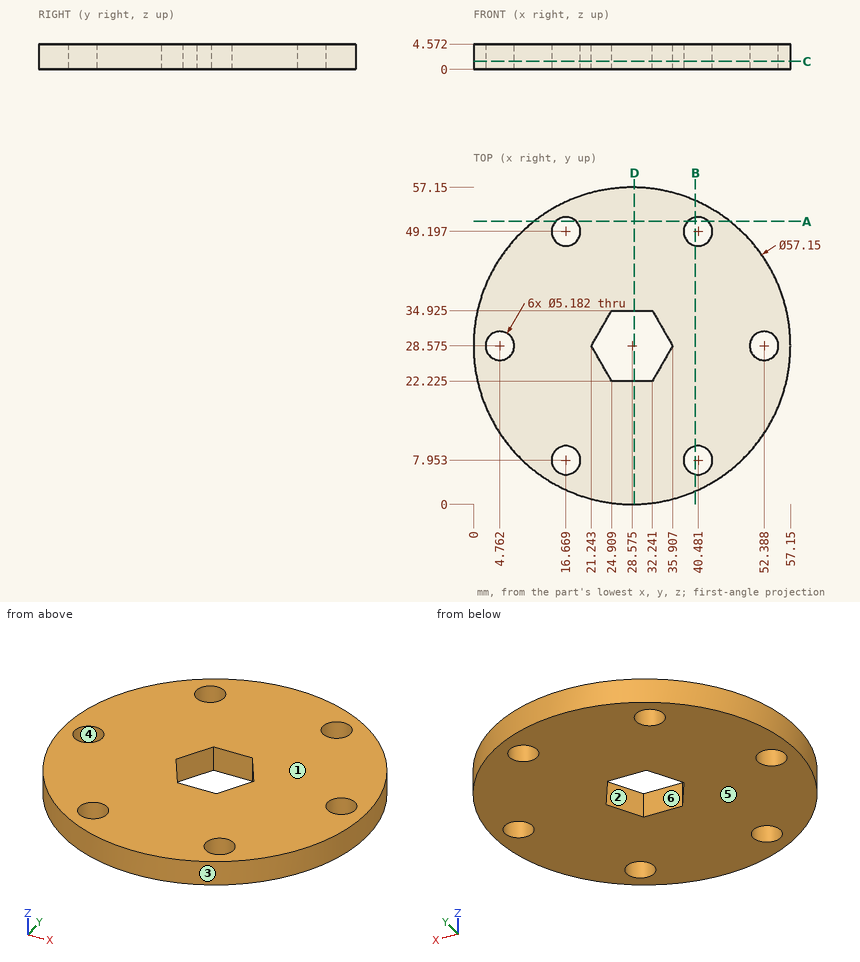
Can you work these out from the drawing? Everything is in mm from the part's minimum corner. A direction names the side the tool comes from. Give positions to 0.01 mm unless a question says otherwise; leave off trailing zeros. Order: outer loops, then holes, each group sorted by start corner. A loop starts at its lowest first (then second) coordinate and runs counter-clockwise, first axis right, second up.
Item 1: If we section it at B-B, the plane x = 40: Write out the boundary of the cut face in (y, z), plus the area to 3 significant figures.
Item 2: If we section it at C-C, the plane z = 1.45: Count the separate pieces of the cut face and the enclosed holes in it, plus the area to 3 significant figures.
Item 3: If we section it at D-D, the plane x = 29: Write out the boundary of the cut face in (y, z) (1 decimal).
Item 4: If we section it at A-A, the plane y = 51: Write out the boundary of the cut face in (x, z) (1 decimal), plus the area to 3 significant figures.
Item 5: For the marked faces 5 and 6, which set-ups out of +Z, -Z, +X, -X, +Y, -Y let a thin tool reach every point of the face, with its end or its side?
Item 6: If we mould it in two halves opening along Y, with no side actions, what happens to the marked faces 1, 2, 3 and 4? For each: pulls with the +Y half, pulls with the -Y half, needs draft (parallel to the pull), parting line crosses it, or undercut.
Item 7: I'm going to push flat-ended pins straight in: pin 1 (1.5 mm diameter, centred on x = 40.5, z = 2.5, fed in from -Y) (1 decimal); pin 2 (3 mm diameter, centred on x = 16.67, y = 49.2, fed in from -Z); pin 3 (1.5 mm diameter, centred on y = 40, z = 3, fed in from +X); pin 4 (1.5 mm diameter, centred on y = 35, z = 4, fed in from -X). Where does each tip first touch, or does it pass through?
Item 8: I need wall thicknesses on line 1 (X direction, y = 47.5, z = 2.25) (1 decimal); line 2 (X direction, y = 50, z = 3.9) (1 decimal); line 3 (X direction, y = 29.5, z = 1.15) (1 decimal). Which ranges of each line are inside material? Lowest first, please.
Values:
1. outline: (2.38, 0) - (5.41, 0) - (5.41, 4.57) - (2.38, 4.57) - close; (10.5, 0) - (46.65, 0) - (46.65, 4.57) - (10.5, 4.57) - close; (51.74, 0) - (54.77, 0) - (54.77, 4.57) - (51.74, 4.57) - close
1. area: 193 mm2
2. separate pieces: 1
2. enclosed holes: 7
2. area: 2,300 mm2
3. outline: (0, 0) - (22.2, 0) - (22.2, 4.6) - (0, 4.6) - close; (34.9, 0) - (57.1, 0) - (57.1, 4.6) - (34.9, 4.6) - close
4. outline: (10.9, 0) - (14.8, 0) - (14.8, 4.6) - (10.9, 4.6) - close; (18.5, 0) - (38.6, 0) - (38.6, 4.6) - (18.5, 4.6) - close; (42.3, 0) - (46.3, 0) - (46.3, 4.6) - (42.3, 4.6) - close
4. area: 128 mm2
5. face 5: -Z, +X, -X, +Y, -Y
5. face 6: +Z, -Z
6. face 1: needs draft
6. face 2: undercut
6. face 3: parting line crosses it
6. face 4: undercut
7. pin 1: stops at y = 2.3
7. pin 2: passes through
7. pin 3: stops at x = 55.08
7. pin 4: stops at x = 0.57
8. line 1: x = 7.2 to 14.7, 18.6 to 38.5, 42.4 to 50
8. line 2: x = 9.7 to 14.2, 19.1 to 38, 42.9 to 47.5
8. line 3: x = 0 to 2.3, 7.2 to 21.8, 35.4 to 50, 54.8 to 57.1
